The listing builds one solid part. Answer for the finished solid, in the listing's coordinates (mm). A direction names the side the tool comes from. Round coordinates to 2 decimals unless told otherwise and drop trailing zeros. Loops run counter-clockwise (first coordinate to the right, second up) from the corner with the lowest first, then second, coordinate; pieces in that order, holes last. Notation, with made-up numbers: (-25.75, -21.5) -> (3.25, -21.5) arc R8 ccw to (3.25, -15.5) -> close; hole circle Ø4 at (79, 36). An arc over 180 degrees is marked (long way). Answer in a Markdown table with one row per item. Add a question column.
```python
from build123d import *

# Parameters (mm, degrees)
EXTRUDE_1_DEPTH     = 15
SKETCH_2_R          = 1.5
CUT_EXTRUDE_1_DEPTH = 34
SKETCH_3_R          = 3
CUT_EXTRUDE_2_DEPTH = 18
CHAMFER_1_SIZE      = 1


with BuildPart() as part:
    # 草图1 → 凸台-拉伸1 (new body)
    with BuildSketch(Plane.XY):
        with BuildLine():
            Line((-21.295, 0), (-10, 0))
            ThreePointArc((-10, 0), (0, -10), (10, 0))
            Line((10, 0), (21.295, 0))
            ThreePointArc((21.295, 0), (0, -21.295), (-21.295, 0))
        make_face()
    extrude(amount=EXTRUDE_1_DEPTH)

    # 草图2 → 切除-拉伸1 (cut)
    with BuildSketch(Plane(origin=(0, 0, 0), x_dir=(1, 0, 0), z_dir=(0, 1, 0))):
        with Locations(Location((-15.6475, -7.5, 0), (0, 0, 270))):
            Circle(SKETCH_2_R)
        with Locations(Location((15.6475, -7.5, 0), (0, 0, 270))):
            Circle(SKETCH_2_R)
    extrude(amount=-CUT_EXTRUDE_1_DEPTH, mode=Mode.SUBTRACT)

    # 草图3 → 切除-拉伸2 (cut)
    with BuildSketch(Plane(origin=(0, -25, 0), x_dir=(1, 0, 0), z_dir=(0, 1, 0))):
        with Locations(Location((-15.6475, -7.5, 0), (0, 0, 90))):
            Circle(SKETCH_3_R)
        with Locations(Location((15.6475, -7.5, 0), (0, 0, 90))):
            Circle(SKETCH_3_R)
    extrude(amount=CUT_EXTRUDE_2_DEPTH, mode=Mode.SUBTRACT)

    # 倒角1
    chamfer_1_edges = [part.edges().sort_by_distance(p)[0] for p in [
        (0, -21.295, 15),
        (0, -21.295, 0),
    ]]
    chamfer(chamfer_1_edges, length=CHAMFER_1_SIZE)


solid = part.part
```
Item 1: Flat-ended cylindrical pins translate along their axes: P1, Ø8, axis at y = -10, z = 6.5, coming from the +X side; P2, Ø2, axis at x = 9, z = 9.5, coming from the -Y side; P3, Ø3, axis at x = -14.5, z = 7.5, coming from the -Y side. Find the tip coordinate at first contact, or state that the pin passes through.
Item 2: Section D-D, the plane z = 2.5 is taken. Write down the section's boundary in (x, y) (3 decimals).
Item 3: Consider L1, parallel to X at y = -4, z = 7.5; L2, parallel to X at y = -13.25, z = 7.5; L3, parallel to Y at x = 14.5, z = 8.75. Determine where each line is inside the solid, lowest interval first. Write a range as from..to.
Item 4: Section A-A, the plane z = 7.5 is taken. Write down the section's boundary in (x, y) (1 decimal), and give its area (3 significant figures).
Item 5: Section C-C, the plane y = -5.5 is taken. Give the number of separate pieces and of enclosed holes in the cut face, and give its area (3 significant figures).
Item 6: Section B-B, the plane x = 0 is taken. Write down the section's boundary in (y, z) (3 decimals), and give its area (3 significant figures).
Item 7: For faces 4 (the cylindrical face through (12.673, -11.011, 7.891)), 5 (the cylindrical face through (0.47, -21.29, 7.41)), determine the directions among +Z, -Z, +X, -X, +Y, -Y from which every point of the face is accessible in a straight line to the end or side of a thin tool.
Item 8: The mould has two halves that part along Z. Classify faces 1 (the flat face through (14, -7, 7)), 2 (the conical face through (0.45, -20.45, 0.16)), 3 (the conical face through (0.45, -20.45, 14.84)): +Z half, -Z half, draft (parallel to the pull), parting line (faces both ways), or undercut.
Here are the results:
| question | item | result |
|---|---|---|
| 1 | P1 | stops at x = 20.43 |
| 1 | P2 | stops at y = -19.74 |
| 1 | P3 | stops at y = -7 |
| 2 | outline | (-21.295, 0) arc R21.295 ccw to (21.295, 0) -> (10, 0) arc R10 cw to (-10, 0) -> close |
| 3 | L1 | x = -20.92..-17.15, -14.15..-9.17, 9.17..14.15, 17.15..20.92 |
| 3 | L2 | x = -12.65..12.65 |
| 3 | L3 | y = -7..0 |
| 4 | outline | (-21.3, 0) arc R21.3 ccw to (-18.6, -10.3) -> (-18.6, -7) -> (-17.1, -7) -> (-17.1, 0) -> close; (-14.1, -7) -> (-12.6, -7) -> (-12.6, -17.1) arc R21.3 ccw to (12.6, -17.1) -> (12.6, -7) -> (14.1, -7) -> (14.1, 0) -> (10, 0) arc R10 cw to (-10, 0) -> (-14.1, 0) -> close; (17.1, -7) -> (18.6, -7) -> (18.6, -10.3) arc R21.3 ccw to (21.3, 0) -> (17.1, 0) -> close |
| 4 | area | 427 mm² |
| 5 | separate pieces | 2 |
| 5 | enclosed holes | 2 |
| 5 | area | 350 mm² |
| 6 | outline | (-21.295, 1) -> (-20.295, 0) -> (-10, 0) -> (-10, 15) -> (-20.295, 15) -> (-21.295, 14) -> close |
| 6 | area | 168 mm² |
| 7 | face 4 | -Y |
| 7 | face 5 | +Z, -Z, -Y |
| 8 | face 1 | undercut |
| 8 | face 2 | -Z half |
| 8 | face 3 | +Z half |
